Can you work these out from the drawing? Everything is in mm from the part's minimum corner. Coordinates: 2 decimals unless noted, no trailing zeros. Order: outer loops, then holes, each group sorted by start corner. A loop starts at its lowest first (then second) coordinate and runs counter-clockwise, first axis right, second up. Notation, with made-up numbers: (56.25, -4) - (112.25, -4) arc R12 ccw to (112.25, 13) - close; hole circle Ø1 at (-21, -22.5). An arc over 180 degrees is marked (long way). Answer as CSV lines item,"result". Start each with the question number.
Item 1: Imagine slicing it at C-C on z = 0.4. List the corners of the cut face in (x, y) for me, and give its area (3 significant figures).
Item 2: I'm going to push a flat-ended pin straight in: pin 1 (2 mm diameter, centred on x = 2.5, y = 5, fed in from -Z). Where does the tip first touch, or does it pass through?
Item 3: I need wall thicknesses on line 1 (Y direction, x = 7.25, z = 2.15); line 2 (Y direction, x = 5.5, z = 0.55); line 3 (Z direction, x = 1.75, y = 6). Which ranges of each line are inside material? Lowest first, please.
Item 4: Imagine slicing it at B-B on x = 9.25. List the corners of the cut face in (y, z) for me.
Item 5: We'd pull the mould along Y, two halves only. Please class the marked faces 1, 2 and 3: pulls with the +Y half, pulls with the -Y half, needs draft (parallel to the pull), parting line crosses it, or undercut.
Item 6: Imagine slicing it at A-A on z = 2.55. List the corners of the cut face in (x, y) for me, and give its area (3 significant figures).
Item 7: Imagine slicing it at D-D on y = 13. List the corners of the cut face in (x, z) for me, and give its area (3 significant figures).
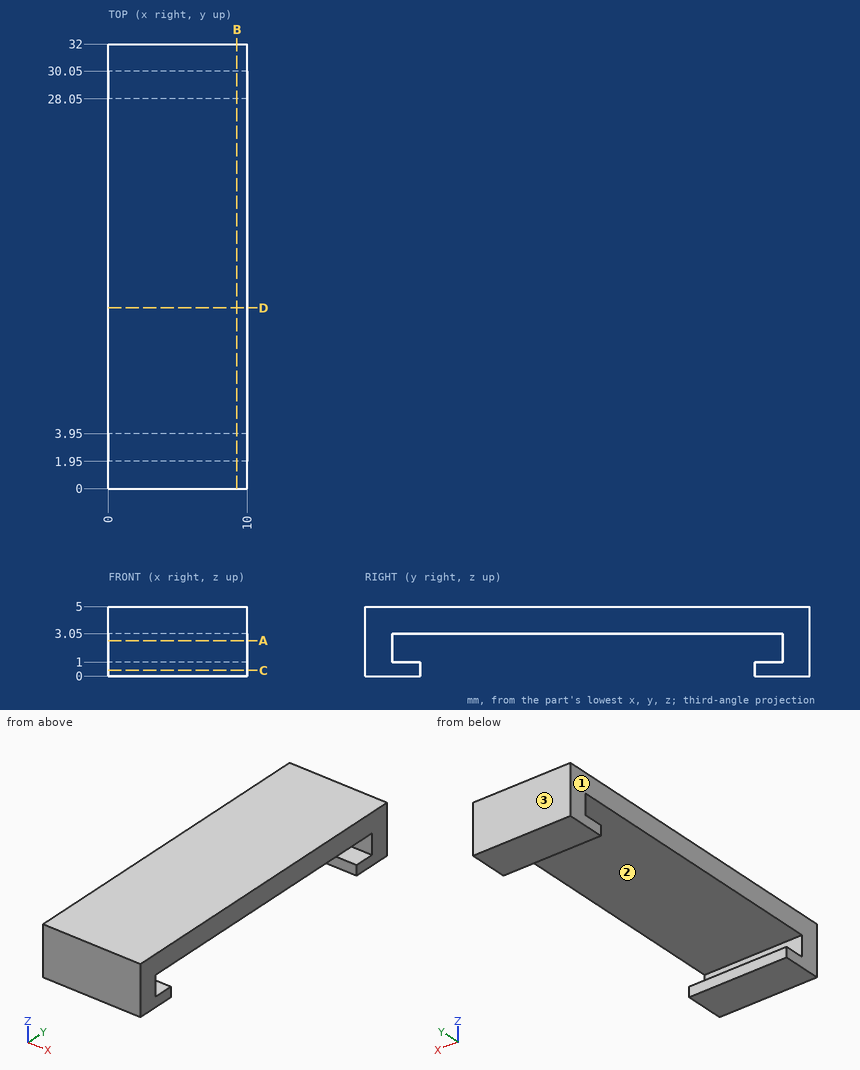
Responses:
1,outline,"(0, 0) - (10, 0) - (10, 3.95) - (0, 3.95) - close; (0, 28.05) - (10, 28.05) - (10, 32) - (0, 32) - close"
1,area,"79.0 mm^2"
2,pin 1,"stops at z = 3.05"
3,line 1,"y = 0 to 1.95, 30.05 to 32"
3,line 2,"y = 0 to 3.95, 28.05 to 32"
3,line 3,"z = 3.05 to 5"
4,outline,"(0, 0) - (3.95, 0) - (3.95, 1) - (1.95, 1) - (1.95, 3.05) - (30.05, 3.05) - (30.05, 1) - (28.05, 1) - (28.05, 0) - (32, 0) - (32, 5) - (0, 5) - close"
5,face 1,"needs draft"
5,face 2,"undercut"
5,face 3,"pulls with the +Y half"
6,outline,"(0, 0) - (10, 0) - (10, 1.95) - (0, 1.95) - close; (0, 30.05) - (10, 30.05) - (10, 32) - (0, 32) - close"
6,area,"39.0 mm^2"
7,outline,"(0, 3.05) - (10, 3.05) - (10, 5) - (0, 5) - close"
7,area,"19.5 mm^2"
